from build123d import *

# Parameters (mm, degrees)
F0_R     = 25.404273
F1_DEPTH = 6.35
F2_W     = 51.59829
F2_H     = 2.908727
F3_DEPTH = 38.1
F5_DEPTH = 51.562
F6_W     = 6.548917
F6_H     = 22.217193
F7_DEPTH = 8.89


with BuildPart() as f1:
    # F0 (on Top) → F1 (new body)
    with BuildSketch(Plane.XY):
        Circle(F0_R)
    extrude(amount=F1_DEPTH)

    # F2 (on face) → F3 (join)
    with BuildSketch(Plane.XY.offset(6.35)):
        with Locations((0.245198, -12.426103)):
            Rectangle(F2_W, F2_H)
    extrude(amount=F3_DEPTH)

    # F4 (on face) → F5 (join)
    with BuildSketch(Plane(origin=(-25.553947, 0, 0), x_dir=(0, -1, 0), z_dir=(-1, 0, 0))):
        Polygon((10.97174, 44.45), (13.880467, 44.45), (-8.800617, 66.449516), (-10.174005, 65.033579), align=None)
    extrude(amount=-F5_DEPTH)

    # F6 (on face) → F7 (join)
    with BuildSketch(Plane.XY.offset(6.35)):
        with Locations((-0.008409, 3.043202)):
            Rectangle(F6_W, F6_H)
    extrude(amount=F7_DEPTH)


solid = f1.part
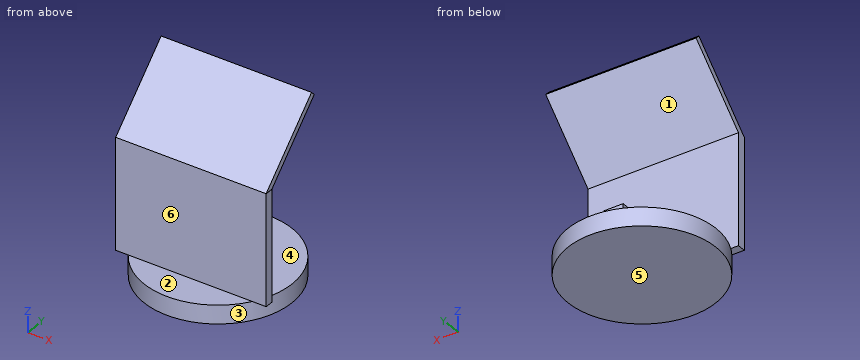
Can you work these out from the model? Positions are in its coordinate system, mm. Face numbers are marked on the shaded views. A direction names the side the tool comes from. Give positions to 0.01 mm unless a question says otherwise; leave off trailing zeros. Loops run counter-clockwise (first coordinate to the right, second up) from the corner with the lowest first, then second, coordinate; pieces in that order, holes last. Notation, with made-up numbers: (36, -30.75) -> (77, -30.75) arc R23 cw to (77, 5.25) -> close; hole circle Ø8 at (-21, -19.5). An arc over 180 degrees is marked (long way). Write item = value, one per line.
1) Suppose I cut it at B-B on y = 0. Write out the boundary of the cut face in (x, z), then the cut area to 3 significant figures.
Check result:
outline = (-25.55, 55.13) -> (26.01, 55.13) -> (26.01, 57.91) -> (-25.55, 57.91) -> close; (-25.4, 0) -> (25.4, 0) -> (25.4, 6.35) -> (3.27, 6.35) -> (3.27, 15.24) -> (-3.28, 15.24) -> (-3.28, 6.35) -> (-25.4, 6.35) -> close
area = 524 mm2
2) Suppose I cut it at A-A on x = 0. Write out the boundary of the cut face in (y, z), then the cut area to 3 significant figures.
Check result:
outline = (-25.4, 0) -> (25.4, 0) -> (25.4, 6.35) -> (14.15, 6.35) -> (14.15, 15.24) -> (-8.07, 15.24) -> (-8.07, 6.35) -> (-10.97, 6.35) -> (-10.97, 44.45) -> (10.17, 65.03) -> (8.8, 66.45) -> (-13.88, 44.45) -> (-13.88, 6.35) -> (-25.4, 6.35) -> close
area = 692 mm2
3) Will these pins go through, and if not, where does the flat tip stop? pin 1 (0.9 mm diameter, centred on x = -23.5, y = -12, fed in from -Z); pin 2 (12 mm diameter, centred on x = -19, y = -16.5, fed in from +Z); pin 3 (4.5 mm diameter, centred on y = 2.5, z = 10, fed in from -X); pin 4 (5 mm diameter, centred on y = -7.5, z = 18, fed in from +X).
Check result:
pin_1 = 6.35
pin_2 = 47.73
pin_3 = -3.28
pin_4 = through
4) Suppose I cut it at D-D on x = 14. Write out the boundary of the cut face in (y, z).
Check result:
outline = (-21.2, 0) -> (21.2, 0) -> (21.2, 6.35) -> (-10.97, 6.35) -> (-10.97, 44.45) -> (10.17, 65.03) -> (8.8, 66.45) -> (-13.88, 44.45) -> (-13.88, 6.35) -> (-21.2, 6.35) -> close
5) I need wall thicknesses on L1, parallel to Y at x = 9, z = 29; L2, parallel to Z at x = -9, y = 11; L3, parallel to Z at x = 7.5, y = -9.5. Which ranges of each line are inside material? Lowest first, please. Write a range as from..to.
Check result:
L1 = -13.88..-10.97
L2 = 0..6.35
L3 = 0..6.35, 45.88..48.7
6) Thinking about a two-plate mould opening in Z: for the marked faces 4, 5 and 6, which applies, released by +Z, released by -Z, zero draft, split by the parting line, or undercut?
Check result:
face_4 = undercut
face_5 = released by -Z
face_6 = zero draft
7) Suppose I cut it at C-C on z = 32.5. Write out the boundary of the cut face in (x, y).
Check result:
outline = (-25.55, -13.88) -> (26.04, -13.88) -> (26.04, -10.97) -> (-25.55, -10.97) -> close
8) For the marked faces 1, 2 and 3, which set-ups out of +Z, -Z, +X, -X, +Y, -Y let a thin tool reach every point of the face, with its end or its side?
Check result:
face_1 = +X, -X, +Y
face_2 = +Z, +X, -X, -Y
face_3 = -Z
